from build123d import *

# Parameters (mm, degrees)
SKETCH_1_R               = 22.5
EXTRUDE_1_DEPTH          = 5
SKETCH_2_R               = 10
EXTRUDE_2_DEPTH          = 5
EXTRUDE_START            = 3
SKETCH_4_R               = 10
EXTRUDE_3_DEPTH          = 3
CUT_EXTRUDE_2_DEPTH      = 35.372954485
CUT_EXTRUDE_2_DEPTH_BACK = 35.372954485
SKETCH_5_R               = 3
HOLE_WIZARD_M4_3_D       = 3.3
SKETCH_10_R              = 1.5
CUT_EXTRUDE_3_DEPTH      = 35.372954485
CHAMFER_2_SIZE           = 0.5
EXTRUDE_START_2          = 5
SKETCH_11_R              = 2
SKETCH_11_R_2            = 1.5
EXTRUDE_4_DEPTH          = 5
CHAMFER_3_SIZE           = 0.5


with BuildPart() as part:
    # 草图1 → 凸台-拉伸1 (new body)
    with BuildSketch(Plane(origin=(0, 0, 0), x_dir=(1, 0, 0), z_dir=(0, 1, 0))):
        with Locations(Location((0, 0, 0), (0, 0, 270))):
            Circle(SKETCH_1_R)
    extrude(amount=EXTRUDE_1_DEPTH)

    # 草图2 → 凸台-拉伸2 (add)
    with BuildSketch(Plane.XZ):
        with Locations(Location((0, 0, 0), (0, 0, 270))):
            Circle(SKETCH_2_R)
    extrude(amount=EXTRUDE_2_DEPTH)

    # 草图4 → 凸台-拉伸3 (add)
    with BuildSketch(Plane(origin=(0, 5, 0), x_dir=(1, 0, 0), z_dir=(0, 1, 0)).offset(EXTRUDE_START)):
        with Locations(Location((0, 0, 0), (0, 0, 90))):
            Circle(SKETCH_4_R)
    extrude(amount=-EXTRUDE_3_DEPTH)

    # 草图5 → 切除-拉伸2 (cut, two sides: drawn at the far end of the back side and taken through both)
    with BuildSketch(Plane(origin=(0, 8, 0), x_dir=(1, 0, 0), z_dir=(0, 1, 0)).offset(-CUT_EXTRUDE_2_DEPTH_BACK)):
        with Locations(Location((0, 0, 0), (0, 0, 270))):
            Circle(SKETCH_5_R)
    extrude(amount=CUT_EXTRUDE_2_DEPTH + CUT_EXTRUDE_2_DEPTH_BACK, mode=Mode.SUBTRACT)

    # M4 螺纹孔3 (through all)
    with Locations(Plane.XZ):
        with Locations((11.913336036, -13.493421527), (13.493421527, 11.913336036), (-11.913336036, 13.493421527), (-13.493421527, -11.913336036)):
            Hole(HOLE_WIZARD_M4_3_D / 2)

    # 草图10 → 切除-拉伸3 (cut, through all)
    with BuildSketch(Plane(origin=(0, 8, 0), x_dir=(1, 0, 0), z_dir=(0, 1, 0))):
        with Locations(Location((0, 6.5, 0), (0, 0, 270))):
            Circle(SKETCH_10_R)
    extrude(amount=-CUT_EXTRUDE_3_DEPTH, mode=Mode.SUBTRACT)

    # 倒角2
    chamfer_2_edges = [part.edges().sort_by_distance(p)[0] for p in [
        (0, 8, -3),
        (0, -5, -3),
    ]]
    chamfer(chamfer_2_edges, length=CHAMFER_2_SIZE)

    # 草图11 → 凸台-拉伸4 (add)
    with BuildSketch(Plane(origin=(0, 8, 0), x_dir=(1, 0, 0), z_dir=(0, 1, 0)).offset(EXTRUDE_START_2)):
        with Locations(Location((0, 6.5, 0), (0, 0, 270))):
            Circle(SKETCH_11_R)
        with Locations(Location((0, 6.5, 0), (0, 0, 270))):
            Circle(SKETCH_11_R_2, mode=Mode.SUBTRACT)
    extrude(amount=-EXTRUDE_4_DEPTH)

    # 倒角3
    chamfer_3_edges = [part.edges().sort_by_distance(p)[0] for p in [
        (0, 13, -8.5),
    ]]
    chamfer(chamfer_3_edges, length=CHAMFER_3_SIZE - 0.0001)  # a hair under: the kernel refuses the full size


solid = part.part
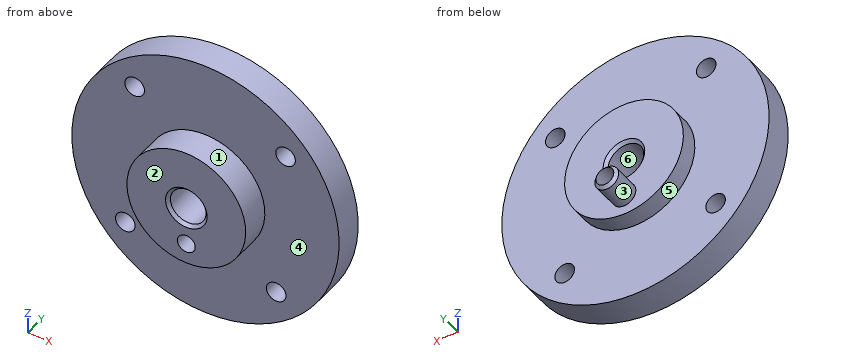
Build history of the part. All positions in model axes, mm. Face numbers are marked on the shaded views. A direction names the side the tool comes from. Coordinates: 2 decimals unless noted, no trailing zeros. Write each loop counter-clockwise with the first axis right and the second up, starting at its lowest first coordinate (ties: lowest second). Pieces come first, ordered by that corner, then holes.
(1) Cut at C-C on y = 9.25. List the corners of the cut face in (x, z), and give its area (3 significant figures).
(2) 3-axis set-ups, long thin cutter, end or side, ignore diameter. For the marked faces 1, 2 and 3: which of +Z, -Z, +X, -X, +Y, -Y reach the whole face in a straight line?
(3) Cut at D-D on y = 3. List the corners of the cut face in (x, z).
(4) Drill centre lines: line 1 (Y direction, x = 4.5, z = -17); line 2 (Z direction, x = 2, y = 7.75); line 3 (X direction, y = 4.75, z = -13). Where is each one in solid material? Low to high.
(5) Cut at A-A on z = 0. List the corners of the cut face in (x, y), and give its area (4 significant figures).
(6) Pin check, flat tips, straight feed: pin 1 Ø2 at (y, z) = (0, -14) entering from +X; pin 2 Ø4.5 at (x, z) = (-13.49, -11.91) entering from +Y; pin 3 Ø4 at (x, z) = (-11.91, 13.49) entering from -Y; pin 4 Ø2 at (x, z) = (11.91, -13.49) entering from -Y. Stop position of each tip, or through.
(7) Cut at B-B on y = 6.75. List the corners of the cut face in (x, z).
(8) Mould opens along Z. For the marked faces 4, 5 and 6 say: pulls with the +Z half, pulls with the -Z half, needs draft (parallel to the pull), parting line crosses it, or undercut.
Working result:
1. outline: circle Ø4 at (0, -6.5); hole circle Ø3 at (0, -6.5)
1. area: 5.50 mm2
2. face 1: -Y
2. face 2: +Z, -Z, +X, -X, -Y
2. face 3: +Y
3. outline: circle Ø45 at (0, 0); hole circle Ø3.3 at (-13.49, -11.91); hole circle Ø3.3 at (-11.91, 13.49); hole circle Ø6 at (0, 0); hole circle Ø3 at (0, -6.5); hole circle Ø3.3 at (11.91, -13.49); hole circle Ø3.3 at (13.49, 11.91)
4. line 1: y = 0 to 5
4. line 2: z = -9.8 to -2.56, 2.56 to 9.8
4. line 3: x = -18.36 to -14.74, -12.25 to 10.34, 13.49 to 18.36
5. outline: (-22.5, 0) - (-10, 0) - (-10, -5) - (-3.5, -5) - (-3, -4.5) - (-3, 7.5) - (-3.5, 8) - (-10, 8) - (-10, 5) - (-22.5, 5) - close; (3, -4.5) - (3.5, -5) - (10, -5) - (10, 0) - (22.5, 0) - (22.5, 5) - (10, 5) - (10, 8) - (3.5, 8) - (3, 7.5) - close
5. area: 306.5 mm2
6. pin 1: stops at x = 18.36
6. pin 2: stops at y = 5
6. pin 3: stops at y = 0
6. pin 4: passes through
7. outline: circle Ø20 at (0, 0); hole circle Ø6 at (0, 0); hole circle Ø3 at (0, -6.5)
8. face 4: needs draft
8. face 5: parting line crosses it
8. face 6: undercut
